Autodesk Inventor part; units mm, degrees
ref_plane "YZ Plane" through (0, 0, 0) normal (1, 0, 0) x (0, 1, 0)
ref_plane "XZ Plane" through (0, 0, 0) normal (0, 1, 0) x (-1, 0, 0)
ref_plane "XY Plane" through (0, 0, 0) normal (0, 0, 1) x (1, 0, 0)
sketch "Sketch1" plane through (0, 0, 0) normal (0, 0, 1) x (1, 0, 0)
  line L0 (0, 78.0122) -> (0, 82.508)
  line L1 (-6.35, 82.508) -> (-6.35, 78.0122)
  line L2 (-6.35, 78.0122) -> (0, 78.0122)
  line L3 (222.25, 130.6664) -> (222.25, 135.1622)
  line L4 (215.9, 135.1622) -> (222.25, 135.1622)
  line L5 (215.9, 135.1622) -> (215.9, 130.6664)
  line L6 (222.25, 77.5379) -> (222.25, 135.1622)
  line L7 (-6.35, 134.6915) -> (-6.35, 78.0122)
  arc A0 (65.1726, 108.6235) -> (63.7223, 104.0872) centre (63.7223, 106.5872) ccw
  line L8 (222.25, 135.1622) -> (104.7076, 135.1622)
  line L9 (22.4128, 134.6915) -> (-6.35, 134.6915)
  line L10 (-6.35, 78.0122) -> (20.7049, 78.0122)
  line L11 (106.4207, 77.5379) -> (222.25, 77.5379)
  arc A1 (104.7076, 135.1622) -> (22.4128, 134.6915) centre (63.7223, 106.5872) ccw
  arc A2 (20.7049, 78.0122) -> (106.4207, 77.5379) centre (63.7223, 106.5872) ccw
  line L12 (215.9, 130.6664) -> (222.25, 130.6664)
  line L13 (0, 82.508) -> (-6.35, 82.508)
  point P0 (0, 0)
extrude "Extrusion1" add sketch "Sketch1" along normal blind 6.35
sketch "Sketch2" plane through (0, 0, 0) normal (0, 0, -1) x (-1, 0, 0)
  line L0 (-53.2456, 114.8496) -> (-74.1989, 114.8496)
  line L1 (-13.716, 122.4622) -> (-13.716, 90.7122)
  line L2 (-63.7223, 114.8496) -> (-63.7223, 83.3208) construction
  line L3 (-13.716, 106.5872) -> (-74.4954, 106.5872) construction
  arc A0 (-63.7223, 109.0872) -> (-61.2223, 106.5872) centre (-63.7223, 106.5872) ccw
  line L4 (-63.7223, 109.0872) -> (-62.2719, 104.5509)
  point P0 (0, 0)
  dimension "d2" = 5
  dimension "d3" = 4.7625
extrude "Extrusion2" cut sketch "Sketch2" against normal through all
sketch "Sketch3" plane through (0, 0, 0) normal (0, 0, -1) x (-1, 0, 0)
  line L0 (6.35, 134.6915) -> (6.35, 78.0122) construction
  line L1 (-222.25, 135.1622) -> (-104.7076, 135.1622) construction
  line L2 (-222.25, 77.5379) -> (-222.25, 135.1622) construction
  line L3 (-106.4207, 77.5379) -> (-222.25, 77.5379) construction
  line L4 (-215.9, 135.1622) -> (-215.9, 130.6664) construction
  line L5 (-217.6131, 96.5879) -> (-200.4173, 96.5879) construction
  line L6 (-200.4173, 90.2379) -> (-217.6131, 90.2379) construction
  line L7 (-217.6131, 90.2379) -> (-217.6131, 96.5879) construction
  line L8 (-217.6131, 121.9879) -> (-200.4173, 121.9879) construction
  line L9 (-200.4173, 115.6379) -> (-217.6131, 115.6379) construction
  line L10 (-217.6131, 115.6379) -> (-217.6131, 121.9879) construction
  circle A0 centre (-219.075, 128.8122) radius 1.8542
  circle A1 centre (-198.5631, 118.8129) radius 1.8542
  line L11 (-222.25, 106.3501) -> (-215.9, 106.3501) construction
  circle A2 centre (-219.075, 83.8879) radius 1.8542
  circle A3 centre (-198.5631, 93.8872) radius 1.8542
  line L12 (-107.95, 135.1622) -> (-107.95, 78.0122) construction
  circle A4 centre (3.175, 128.8122) radius 1.8542
  circle A5 centre (-17.3369, 118.8129) radius 1.8542
  circle A6 centre (-17.3369, 93.8872) radius 1.8542
  circle A7 centre (3.175, 83.8879) radius 1.8542
  line L13 (-200.4173, 121.9879) -> (-200.4173, 115.6379)
  line L14 (-200.4173, 96.5879) -> (-200.4173, 90.2379)
  point P0 (0, 0)
  point P1 (-215.9, 135.1622)
  dimension "d7" = 3.7084
  dimension "d8" = 3.175
  dimension "d9" = 3.175
  dimension "d10" = 6.35
  dimension "d11" = 3.7084
  dimension "d12" = 19.05
  dimension "d13" = 28.8121
  dimension "d14" = 28.8121
  dimension "d15" = 114.3
  dimension "d16" = 114.3
extrude "Extrusion3" cut sketch "Sketch3" against normal through all
equation "\"d8\" = d9"
equation "\"d13\" = d14"
equation "\"d15\" = d16"
properties part number "tiltStructureCrossBeam" material "Wood (Cherry)"
For this review, take the finished solid that the model builds, in its own axes (mm). A direction names the side the tool comes from. Round coordinates to 2 decimals unless told otherwise and drop trailing zeros. Write each loop counter-clockwise with the first axis right and the second up, starting at its lowest first coordinate (ties: lowest second). Pieces come first, ordered by that corner, then holes.
1) For line 1 along X through (y, z) = (84, 3.75); line 2 along X through (y, z) = (120.5, 0.75); line 3 along Y through (x, z) = (174, 5.5), list the stretches that pass through material, from the lowest coordinate up.
Answer below:
line 1: x = -6.35 to -5.03, -1.32 to 217.22, 220.93 to 222.25
line 2: x = -6.35 to 16.57, 18.11 to 197.79, 199.33 to 222.25
line 3: y = 77.54 to 135.16
2) Machinability: for faces 1 (the face through (7, 78.012, 3)), 2 (the face through (106, 106, 6.35)), 3 (the face through (164, 77.538, 3)), 4 (the face through (63.007, 106.851, 3.131)), 5 (the face through (164, 135.162, 3)), which of the approach directions +Z, -Z, +X, -X, +Y, -Y give a long, thin tool a straight path to every point of the face, cutting with its end or side? Answer none if there is none.
Answer below:
face 1: +Z, -Z, -X, -Y
face 2: +Z, +X, -X, +Y, -Y
face 3: +Z, -Z, +X, -Y
face 4: +Z, -Z
face 5: +Z, -Z, +X, +Y
3) Take a section at B-B on y = 64. Give the boundary of the cut face in (x, z), then the cut area to 3 significant figures.
Answer below:
outline: (34.51, 0) - (92.93, 0) - (92.93, 6.35) - (34.51, 6.35) - close
area: 371 mm2
4) Take a section at C-C on x = 79.5. Give the boundary of the cut face in (y, z).
Answer below:
outline: (57.41, 0) - (153.99, 0) - (153.99, 6.35) - (57.41, 6.35) - close
5) Insertion check: pin 1 Ø3 at (x, z) = (172.5, 2.5) entering from -Y; pin 2 Ø4.5 at (x, y) = (198.56, 93.89) entering from +Z; pin 3 Ø2 at (x, z) = (30, 3) entering from -Y; pin 4 Ø1.5 at (y, z) = (140.5, 4) entering from +X. Each pin has a flat end and moves straight along its axis. Give the tip position at first contact, or say it passes through.
Answer below:
pin 1: stops at y = 77.54
pin 2: stops at z = 6.35
pin 3: stops at y = 66.63
pin 4: stops at x = 101.09
6) Mouldability with a two-part tool opening along Y and no side actions: class faces 6 (the face through (66.123, 105.889, 3.131)), 7 (the face through (8, 134.692, 3)), 8 (the face through (106, 106, 0)) as +Y half, -Y half, draft (parallel to the pull), parting line (faces both ways), or undercut.
Answer below:
face 6: undercut
face 7: +Y half
face 8: draft
7) Take a section at A-A on z = 2.75. State how many separate pieces and enclosed holes the cut face has, then the cut area to 3 significant figures.
Answer below:
separate pieces: 1
enclosed holes: 9
area: 15,600 mm2
